Could you check a few things on this drawing? It's one solid part, dimensions in mm from its lowest x, y, z. A direction names the side the tool comes from. Round coordinates to 2 decimals unless told otherwise and drop trailing zeros. Write each loop counter-clockwise with the first axis right and the second up, starting at its lowest first coordinate (ties: lowest second). Pieces come first, ordered by that corner, then holes. Notation, with made-up numbers: (19.25, 47.5) -> (40.25, 47.5) arc R24 ccw to (40.25, 80.5) -> close; hole circle Ø11 at (2.5, 30). An arc over 180 degrees is marked (long way). Put each result on its own line as item: value. Start each with the question number.
1) Will this pin go through, and if not, where does the flat tip stop? P1, Ø2.5, axis at x = 27.375, y = 8.82, coming from the -Z side.
2) Which directions (+Z, -Z, +X, -X, +Y, -Y) give clear straight access to the entire face, cutting with the end or side of a thin tool? Please do the marked faces 4 and 5.
3) I want a section at A-A, the plane y = 8.82. List the corners of the cut face in (x, z) for me (3 decimals), then the cut area to 3 significant figures.
4) I want a section at B-B, the plane y = 5. List the corners of the cut face in (x, z) for me, then the cut area to 3 significant figures.
5) I want a section at C-C, the plane z = 1.7. List the corners of the cut face in (x, y) for me (3 decimals), then the cut area to 3 significant figures.
6) If I drill on line 1 along X through (y, z) = (6.25, 3.7); line 2 along X through (y, z) = (10.5, 1.7); line 3 along X through (y, z) = (8.5, 1.6), over which ranges is the centre line in solid material (lowest first)? Write a range as [from, to].
7) We'd pull the mould along Y, two halves only. Please class the marked faces 1, 2 and 3: released by +Y, released by -Y, zero draft, split by the parting line, or undercut.
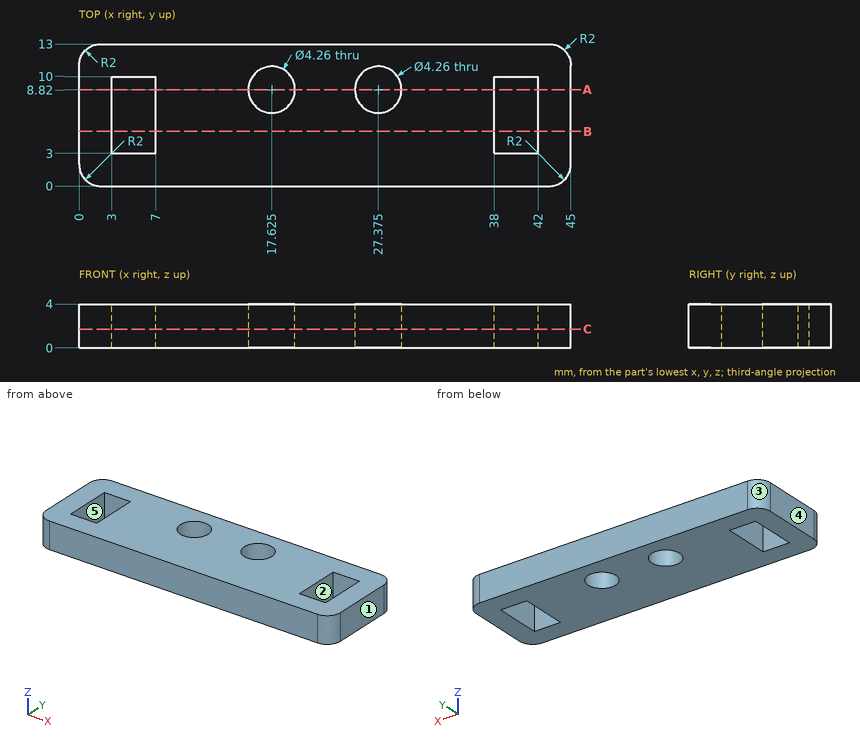
Findings:
1. P1: passes through
2. face 4: +Z, -Z, -X, +Y, -Y
2. face 5: +Z, -Z
3. outline: (0, 0) -> (3, 0) -> (3, 4) -> (0, 4) -> close; (7, 0) -> (15.495, 0) -> (15.495, 4) -> (7, 4) -> close; (19.755, 0) -> (25.245, 0) -> (25.245, 4) -> (19.755, 4) -> close; (29.505, 0) -> (38, 0) -> (38, 4) -> (29.505, 4) -> close; (42, 0) -> (45, 0) -> (45, 4) -> (42, 4) -> close
3. area: 114 mm2
4. outline: (0, 0) -> (3, 0) -> (3, 4) -> (0, 4) -> close; (7, 0) -> (38, 0) -> (38, 4) -> (7, 4) -> close; (42, 0) -> (45, 0) -> (45, 4) -> (42, 4) -> close
4. area: 148 mm2
5. outline: (0, 2) arc R2 ccw to (2, 0) -> (43, 0) arc R2 ccw to (45, 2) -> (45, 11) arc R2 ccw to (43, 13) -> (2, 13) arc R2 ccw to (0, 11) -> close; hole (3, 3) -> (7, 3) -> (7, 10) -> (3, 10) -> close; hole circle Ø4.26 at (17.625, 8.82); hole circle Ø4.26 at (27.375, 8.82); hole (38, 3) -> (42, 3) -> (42, 10) -> (38, 10) -> close
5. area: 497 mm2
6. line 1: x = [0, 3], [7, 38], [42, 45]
6. line 2: x = [0, 16.32], [18.93, 26.07], [28.68, 45]
6. line 3: x = [0, 3], [7, 15.52], [19.73, 25.27], [29.48, 38], [42, 45]
7. face 1: zero draft
7. face 2: undercut
7. face 3: released by +Y
